Input: dimensioned drawing with shaded views. Units: mm. Origin: part minimum x, y, z. Round coordinates to 2 decimals unless told otherwise and drop trailing zeros. Loops run counter-clockwise (first coordinate to the right, second up) from the corner with the lowest first, then second, coordinate; pieces in that order, holes last. Notation, with made-up numbers: M 18.25,86 L 64.25,86 A18 ccw 64.25,120 Z; hole C -28.75,-6.75 d9. An arc over 180 degrees is marked long. Write each question's results on one line, items separated by ' | '. Start each with the question number.
1. Section A-A on y = 4. Output: boundary loops of the cut face in (x, z).
2. Ray query, line 1 (Y direction, x = 10.5, z = 0.1) (1 decimal); line 2 (X direction, y = 1.5, z = 0.1); line 3 (Z direction, x = 3, y = 6.5). Return the intervals inside material, ascending.
3. Section C-C on x = 3.5. Output: boundary loops of the cut face in (y, z).
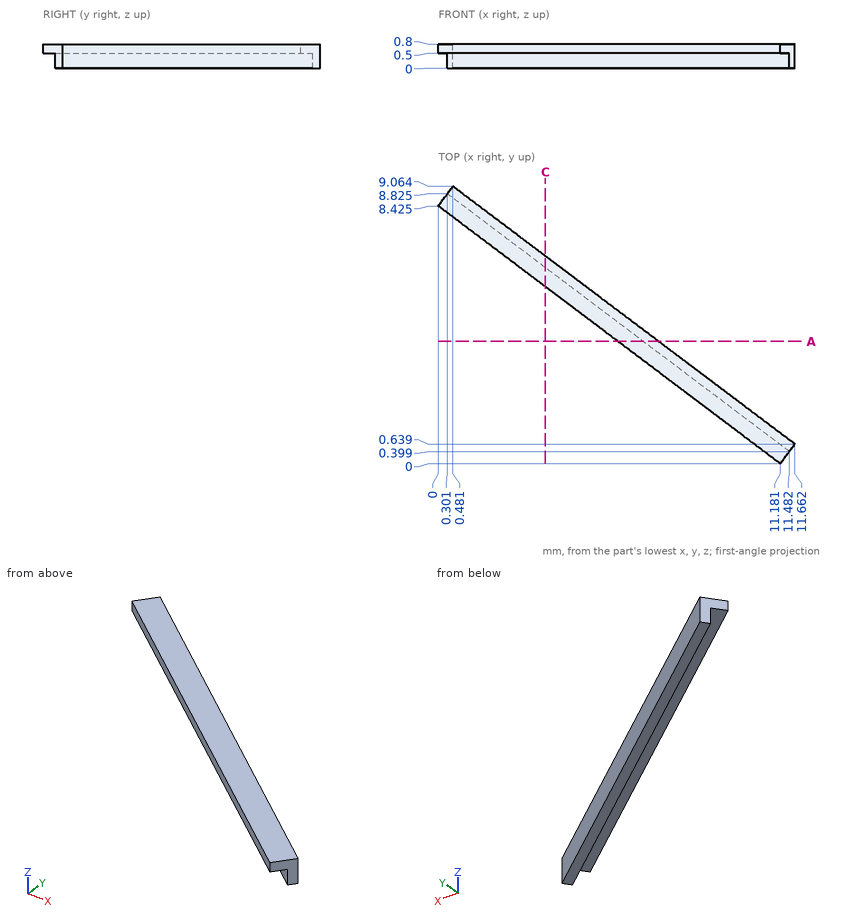
Taken from the geometry:
1) outline: M 5.87,0.5 L 6.7,0.5 L 6.7,0 L 7.2,0 L 7.2,0.8 L 5.87,0.8 Z
2) line 1: 1.1 to 1.5 | line 2: 10.02 to 10.52 | line 3: 0.5 to 0.8
3) outline: M 5.79,0.5 L 6.41,0.5 L 6.41,0 L 6.79,0 L 6.79,0.8 L 5.79,0.8 Z
